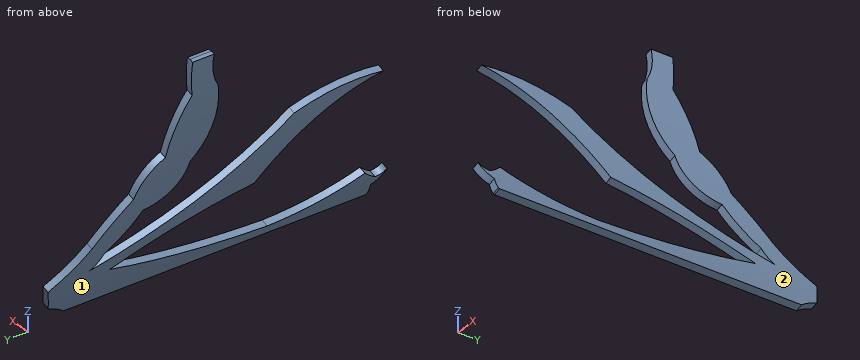
from build123d import *

# Parameters (mm, degrees)
BASE_FLANGE1_DEPTH = 152.4
CUT_EXTRUDE2_DEPTH = 210.453765781
SKETCH8_OUTSIDE_W  = 91.669
SKETCH8_OUTSIDE_H  = 186.952
CUT_EXTRUDE3_DEPTH = 156.159268245
CUT_EXTRUDE5_DEPTH = 150.529804304
CUT_EXTRUDE6_DEPTH = 150.529804304


# Sheet-metal steps are written as plain solids
with BuildPart() as part:
    # Sketch1 → Base-Flange1 (new body)
    with BuildSketch(Plane(origin=(0, 0, 0), x_dir=(1, 0, 0), z_dir=(0, 1, 0))):
        with BuildLine():
            ThreePointArc((101.6, 0), (0, 101.6), (-101.6, 0))
            Line((-101.6, 0), (-100.076, 0))
            ThreePointArc((-100.076, 0), (0, 100.076), (100.076, 0))
            Line((100.076, 0), (101.6, 0))
        make_face()
    extrude(amount=BASE_FLANGE1_DEPTH)

    # Sketch7 → Cut-Extrude2 (cut, through all)
    with BuildSketch(Plane(origin=(0, 0, 0), x_dir=(1, 0, 0), z_dir=(0, 1, 0))):
        Polygon((-91.709043777, 57.490350595), (138.01260718, -58.815220223), (145.858691999, 79.364012989), (-90.642426647, 185.885465098), align=None)
    extrude(amount=CUT_EXTRUDE2_DEPTH, mode=Mode.SUBTRACT)

    # Sketch8 outside → Cut-Extrude3 (cut, through all)
    with BuildSketch(Plane(origin=(-92.234633035, 0, -26.893225996), x_dir=(-0.27991806035793976, 0, 0.9600238952679506), z_dir=(-0.9600238952679506, 0, -0.27991806035793976))):
        with Locations((-0.1185, 76.2)):
            Rectangle(SKETCH8_OUTSIDE_W, SKETCH8_OUTSIDE_H)
        with BuildLine():
            Line((28.228420724, 123.255255295), (28.228420724, 63.013426534))
            Line((28.228420724, 63.013426534), (-23.710305665, 67.943144138))
            Line((-23.710305665, 67.943144138), (-24.773491826, 75.417539706))
            Line((-24.773491826, 75.417539706), (-24.773491826, 140.385814226))
            ThreePointArc((-24.773491826, 140.385814226), (-22.985555805, 142.451644443), (-21.54666964, 144.774137995))
            Line((-21.54666964, 144.774137995), (-15.477635794, 146.793089403))
            ThreePointArc((-15.477635794, 146.793089403), (-11.468978559, 143.067294692), (-6.985554285, 139.928857844))
            ThreePointArc((-6.985554285, 139.928857844), (-2.02114191, 136.922848828), (2.45774455, 133.232177276))
            ThreePointArc((2.45774455, 133.232177276), (6.806375414, 131.32724859), (9.926241691, 127.748732402))
            ThreePointArc((9.926241691, 127.748732402), (16.039086335, 126.228175305), (21.554569405, 123.185411754))
            ThreePointArc((21.554569405, 123.185411754), (24.888843169, 123.473733589), (28.228420724, 123.255255295))
        make_face(mode=Mode.SUBTRACT)
    extrude(amount=CUT_EXTRUDE3_DEPTH, mode=Mode.SUBTRACT)

    # Sketch9 → Cut-Extrude5 (cut, through all)
    with BuildSketch(Plane(origin=(-92.234633035, 0, -26.893225996), x_dir=(-0.27991806035793976, 0, 0.9600238952679506), z_dir=(-0.9600238952679506, 0, -0.27991806035793976))):
        with BuildLine():
            Line((-24.501828907, 76.777557676), (-27.569176237, 78.5320759))
            Line((-27.569176237, 78.5320759), (-29.494089624, 68.863518536))
            Line((-29.494089624, 68.863518536), (-21.26675398, 50.764523355))
            Line((-21.26675398, 50.764523355), (28.228420724, 57.34408301))
            Line((28.228420724, 57.34408301), (28.013079808, 118.763565618))
            ThreePointArc((28.013079808, 118.763565618), (24.75429403, 118.880140281), (21.705230571, 117.724075223))
            ThreePointArc((21.705230571, 117.724075223), (13.693303318, 118.137203319), (6.704304858, 122.076182077))
            ThreePointArc((6.704304858, 122.076182077), (1.166010219, 124.850428459), (-1.395339362, 130.490343247))
            ThreePointArc((-1.395339362, 130.490343247), (-5.917319527, 133.265505392), (-9.991337743, 136.664358893))
            ThreePointArc((-9.991337743, 136.664358893), (-11.942393165, 137.4181864), (-13.626649766, 138.658409311))
            ThreePointArc((-13.626649766, 138.658409311), (-4.330180004, 118.477783543), (8.758521079, 100.523176602))
            ThreePointArc((8.758521079, 100.523176602), (10.931974112, 91.396763407), (10.672272602, 82.018710783))
            ThreePointArc((10.672272602, 82.018710783), (5.176812074, 95.990549965), (-5.917317854, 106.106510507))
            ThreePointArc((-5.917317854, 106.106510507), (-9.582838682, 120.389201142), (-15.747934485, 133.784084063))
            ThreePointArc((-15.747934485, 133.784084063), (-20.011123577, 116.370294996), (-22.090885373, 98.563290146))
            ThreePointArc((-22.090885373, 98.563290146), (-20.494324779, 88.872234651), (-16.433576157, 79.929311026))
            ThreePointArc((-16.433576157, 79.929311026), (-17.84229029, 78.509895577), (-19.097539053, 76.953114838))
            ThreePointArc((-19.097539053, 76.953114838), (-18.740022488, 75.714547524), (-17.763603379, 74.872839255))
            ThreePointArc((-17.763603379, 74.872839255), (-19.832219816, 75.585249002), (-21.44191431, 77.066999739))
            ThreePointArc((-21.44191431, 77.066999739), (-22.961230073, 76.809778861), (-24.501828907, 76.777557676))
        make_face()
    extrude(amount=CUT_EXTRUDE5_DEPTH, mode=Mode.SUBTRACT)

    # Sketch10 → Cut-Extrude6 (cut, through all)
    with BuildSketch(Plane(origin=(-92.234633035, 0, -26.893225996), x_dir=(-0.27991806035793976, 0, 0.9600238952679506), z_dir=(-0.9600238952679506, 0, -0.27991806035793976))):
        Polygon((28.013079808, 118.763565618), (28.728121694, 118.655926759), (28.728121694, 52.453532496), (22.818416534, 52.453532496), (26.943491202, 118.763565618), align=None)
    extrude(amount=CUT_EXTRUDE6_DEPTH, mode=Mode.SUBTRACT)


solid = part.part
Part model, mm, in its own coordinate system. Face numbers are marked on the shaded views. Round coordinates to 2 decimals unless told otherwise and drop trailing zeros. Loops run counter-clockwise (first coordinate to the right, second up) from the corner with the lowest first, then second, coordinate; pieces in that order, holes last. Notation, with made-up numbers: (83, 3.25) - (123, 3.25) arc R8 ccw to (123, 17.25) - close; hole circle Ø8 at (58.5, 79). An arc over 180 degrees is marked (long way). Answer as a JSON object with one key per item and string values.
Item 1: Wall check: L1, parallel to Z at x = -89, y = 124; L2, parallel to Z at x = -99.5, y = 87.5; L3, parallel to X at y = 126, z = -46.5. Give the ranges that are in metal, low to high.
Output:
{"L1": "-49.01 to -45.76", "L2": "-19.24 to -17.43", "L3": "-90.33 to -88.62"}
Item 2: Pull direction Z, two halves, no side cores. Call the marked faces 1 and 2: pulls with the +Z half, pulls with the -Z half, needs draft (parallel to the pull), parting line crosses it, or undercut.
Output:
{"face 1": "pulls with the -Z half", "face 2": "pulls with the +Z half"}
Item 3: Pin check, flat tips, straight feed: pin 1 (1 mm diameter, centred on y = 119.5, z = -34, fed in from +X); pin 2 (2 mm diameter, centred on y = 126.5, z = -26.5, fed in from -X); pin 3 (2 mm diameter, centred on x = -95, y = 124, fed in from -Z). Stop position of each tip, or through.
Output:
{"pin 1": "x = -93.94", "pin 2": "x = -98.35", "pin 3": "z = -38.56"}
Item 4: Band-saw the part on B-B on y = 109. List the corners of the cut face in (x, z).
Output:
{"outline": "(-98.05, -26.61) arc R101.6 ccw to (-95.54, -34.57) - (-94.07, -34.14) arc R100.08 cw to (-96.59, -26.19) - close; (-89.48, -48.12) arc R101.6 ccw to (-87.66, -51.36) - (-86.15, -50.92) arc R100.08 cw to (-87.99, -47.68) - close"}
Item 5: Band-saw the part on C-C on y = 142.5. List the corners of the cut face in (x, z).
Output:
{"outline": "(-93.98, -38.6) arc R101.6 ccw to (-88.59, -49.74) - (-87.09, -49.3) arc R100.08 cw to (-92.51, -38.17) - close"}
Item 6: Band-saw the part on A-A on y = 89.5. List the corners of the cut face in (x, z), plus the area to 3 significant figures.
Output:
{"outline": "(-100.06, -17.64) arc R101.6 ccw to (-99.61, -20.03) - (-98.14, -19.6) arc R100.08 cw to (-98.59, -17.21) - close; (-89.71, -47.7) arc R101.6 ccw to (-87.66, -51.36) - (-86.15, -50.92) arc R100.08 cw to (-88.21, -47.26) - close", "area": "10.1 mm2"}
